Geometry: final body of the model. Coordinates: model frame, mm. A direction names the side the tool comes from. Round coordinates to 2 decimals unless told otherwise and drop trailing zeros. Write each loop counter-clockwise with the first axis right and the second up, starting at its lowest first coordinate (ties: lowest second). Pieces come first, ordered by that corner, then holes. Notation, with made-up numbers: (70.25, 57.25) -> (102.25, 57.25) arc R29 ccw to (102.25, 94.25) -> close; hole circle Ø1 at (57, -38). An arc over 180 degrees is marked (long way). One line per item, written item: value. Start each with the question number.
from build123d import *

# Parameters (mm, degrees)
SKETCH_1_W          = 200
SKETCH_1_H          = 140
SKETCH_1_R          = 3.25
EXTRUDE_1_DEPTH     = 5
FILLET_1_R          = 20
SKETCH_3_W          = 5
SKETCH_3_H          = 30
CUT_EXTRUDE_1_DEPTH = 39


with BuildPart() as part:
    # 草图1 → 凸台-拉伸1 (new body)
    with BuildSketch(Plane.XY):
        with Locations((0, 50)):
            Rectangle(SKETCH_1_W, SKETCH_1_H)
        with Locations((30, 80)):
            Circle(SKETCH_1_R, mode=Mode.SUBTRACT)
        with Locations(Location((30, 20, 0), (0, 0, 180))):
            Circle(SKETCH_1_R, mode=Mode.SUBTRACT)
        with Locations(Location((-30, 80, 0), (0, 0, 180))):
            Circle(SKETCH_1_R, mode=Mode.SUBTRACT)
        with Locations((-30, 20)):
            Circle(SKETCH_1_R, mode=Mode.SUBTRACT)
    extrude(amount=EXTRUDE_1_DEPTH)

    # 圆角1
    fillet_1_edges = [part.edges().sort_by_distance(p)[0] for p in [
        (-100, 120, 2.5),
        (-100, -20, 2.5),
        (100, -20, 2.5),
        (100, 120, 2.5),
    ]]
    fillet(fillet_1_edges, radius=FILLET_1_R)

    # 草图3 → 切除-拉伸1 (cut)
    with BuildSketch(Plane.XY.offset(5)):
        with Locations((97.5, 75)):
            Rectangle(SKETCH_3_W, SKETCH_3_H)
        with Locations((97.5, 30)):
            Rectangle(SKETCH_3_W, SKETCH_3_H)
        with Locations((-97.5, 30)):
            Rectangle(SKETCH_3_W, SKETCH_3_H)
        with Locations((-97.5, 75)):
            Rectangle(SKETCH_3_W, SKETCH_3_H)
    extrude(amount=-CUT_EXTRUDE_1_DEPTH, mode=Mode.SUBTRACT)


solid = part.part
(1) Section query C-C (x = 30). Output: boundary loops of the cut face in (y, z), and give its area (3 significant figures).
(2) Line query: probe 1 along Y at (x, z) = (-30, 1.55); probe 2 along X at (y, z) = (89.5, 1.2); probe 3 along X at (y, z) = (-6, 4). Output: solid intervals per line, ascending.
(3) Section query B-B (z = 2.45). Output: boundary loops of the cut face in (x, y).
(4) Set-up query: faces 1 (the face through (-1, 120, 2)), 2 (the face through (97, 45, 3)), 3 (the face through (-98, 15, 3)). Return all of +Z, -Z, +X, -X, +Y, -Y with unobstructed straight access to the full face (end or side cutting, diameter ignored); none if empty.
(5) Pin query (flat end, axial travel): pin 1 (2.5 mm diameter, centred on x = 97.5, z = 3, fed in from -Y); pin 2 (1.5 mm diameter, centred on y = 68, z = 3.5, fed in from -X); pin 3 (8.5 mm diameter, centred on x = -30, y = 20, fed in from -Z); pin 4 (1.5 mm diameter, centred on x = -98, z = 1.5, fed in from -Y). Return the tip coordinate at first contact, or that it passes through.
(6) Section query A-A (y = 20). Output: boundary loops of the cut face in (x, z), and give its area (3 significant figures).
(7) Pull-direction query (X, two-part tool) for faces 4 (the face through (-95, 75, 3)), 5 (the face through (-31.5, 82.883, 2.465)), 6 (the face through (31.5, 77.117, 2.465)), 7 (the face through (95, 75, 3)); classes: pulls with the +X half, pulls with the -X half, needs draft (parallel to the pull), parting line crosses it, or undercut.
(8) Section query D-D (y = 39.5). Output: boundary loops of the cut face in (x, z).
Results list:
1. outline: (-20, 0) -> (16.75, 0) -> (16.75, 5) -> (-20, 5) -> close; (23.25, 0) -> (76.75, 0) -> (76.75, 5) -> (23.25, 5) -> close; (83.25, 0) -> (120, 0) -> (120, 5) -> (83.25, 5) -> close
1. area: 635 mm^2
2. probe 1: y = -20 to 16.75, 23.25 to 76.75, 83.25 to 120
2. probe 2: x = -95 to 95
2. probe 3: x = -99.08 to 99.08
3. outline: (-100, 0) arc R20 ccw to (-80, -20) -> (80, -20) arc R20 ccw to (100, 0) -> (100, 15) -> (95, 15) -> (95, 45) -> (100, 45) -> (100, 60) -> (95, 60) -> (95, 90) -> (100, 90) -> (100, 100) arc R20 ccw to (80, 120) -> (-80, 120) arc R20 ccw to (-100, 100) -> (-100, 90) -> (-95, 90) -> (-95, 60) -> (-100, 60) -> (-100, 45) -> (-95, 45) -> (-95, 15) -> (-100, 15) -> close; hole circle Ø6.5 at (-30, 20); hole circle Ø6.5 at (-30, 80); hole circle Ø6.5 at (30, 20); hole circle Ø6.5 at (30, 80)
4. face 1: +Z, -Z, +X, -X, +Y
4. face 2: +Z, -Z, +X
4. face 3: +Z, -Z, -X
5. pin 1: stops at y = -11.66
5. pin 2: stops at x = -95
5. pin 3: stops at z = 0
5. pin 4: stops at y = -10.12
6. outline: (-95, 0) -> (-33.25, 0) -> (-33.25, 5) -> (-95, 5) -> close; (-26.75, 0) -> (26.75, 0) -> (26.75, 5) -> (-26.75, 5) -> close; (33.25, 0) -> (95, 0) -> (95, 5) -> (33.25, 5) -> close
6. area: 885 mm^2
7. face 4: pulls with the -X half
7. face 5: undercut
7. face 6: undercut
7. face 7: pulls with the +X half
8. outline: (-95, 0) -> (95, 0) -> (95, 5) -> (-95, 5) -> close
